Source: CAD feature listing. Evaluate the final solid. Frame: model axes, mm. A direction names the side the tool comes from. Give positions to 0.01 mm unless a question says otherwise; leave off trailing zeros. Write each loop counter-clockwise with the first axis right and the second up, starting at its lowest first coordinate (ties: lowest second). Pieces come first, ordered by that corner, then holes.
```python
from build123d import *

# Parameters (mm, degrees)
F0_W        = 615
F0_H        = 1035
F1_DEPTH    = 436
F2_W        = 383.7750256062
F2_H        = 30
F2_W_2      = 88.2078781724
F3_DEPTH    = 10
F4_W        = 436
F4_H        = 368.6535954475
F5_DEPTH    = 43
F6_T4_DEPTH = 436
F6_T9_DEPTH = 436
F7_W        = 102.6465103626
F7_H        = 30
F7_W_2      = 88.2078781724
F8_DEPTH    = 51
F9_W        = 30
F9_H        = 30
F10_DEPTH   = 55
F11_W       = 30
F11_H       = 30
F12_DEPTH   = 100
F14_DEPTH   = 30
F15_W       = 53
F15_H       = 27.2612595558
F16_DEPTH   = 57
F17_W       = 67.928535223
F17_H       = 25.3568291664
F18_DEPTH   = 81
F20_DEPTH   = 30
F22_DEPTH   = 25


# Not quite as in the source:
# - a fillet or chamfer that OpenCascade refuses, or shapes differently, is made with other operations: its cross-section is extruded or revolved along the edge and cut away or added


with BuildPart() as f1:
    # F0 (on Front) → F1 (new body)
    with BuildSketch(Plane.XZ):
        with Locations((0, 517.5)):
            Rectangle(F0_W, F0_H)
        Polygon((227.5, 80), (-227.5, 80), (-227.5, 360), (-257.5, 360), (-257.5, 440), (-227.5, 440), (-227.5, 520), (-257.5, 520), (-257.5, 665), (-227.5, 665), (-227.5, 955), (227.5, 955), (227.5, 665), (267.5, 665), (297.5, 665), (297.5, 635), (267.5, 635), (267.5, 550), (297.5, 550), (297.5, 520), (267.5, 520), (227.5, 520), (227.5, 440), (297.5, 440), (297.5, 360), (227.5, 360), align=None, mode=Mode.SUBTRACT)
    extrude(amount=F1_DEPTH)

    # F2 (on face) → F3 (cut, through all)
    with BuildSketch(Plane.YZ.offset(307.5)):
        with Locations((-191.8875128031, 535)):
            Rectangle(F2_W, F2_H)
        with Locations((-44.1039390862, 650)):
            Rectangle(F2_W_2, F2_H)
    extrude(amount=-F3_DEPTH, mode=Mode.SUBTRACT)

    # F4 (on face) → F5 (join)
    with BuildSketch(Plane.YZ.offset(307.5)):
        with Locations((-218, 525.7607400417)):
            Rectangle(F4_W, F4_H)
    extrude(amount=F5_DEPTH)

    # F6: chamfer of 45 on 2 edges, made by hand


with BuildPart() as f6_tool2:
    # F6_s3 → F6_t4 (new body)
    with BuildSketch(Plane.XZ):
        Polygon((307.5, 755.0875377655), (352.5, 710.0875377655), (307.5, 710.0875377655), align=None)
    extrude(amount=F6_T4_DEPTH)

    split(bisect_by=Plane.YZ.offset(350.5), keep=Keep.BOTTOM)


with BuildPart() as f1_1:
    add(f1.part)

    # F6_t1: union F6_tool2
    add(f6_tool2.part)


with BuildPart() as f6_tool7:
    # F6_s8 → F6_t9 (new body)
    with BuildSketch(Plane.XZ.offset(436)):
        Polygon((307.5, 296.433942318), (352.5, 341.433942318), (307.5, 341.433942318), align=None)
    extrude(amount=-F6_T9_DEPTH)

    split(bisect_by=Plane.YZ.offset(350.5), keep=Keep.BOTTOM)


with BuildPart() as f1_2:
    add(f1_1.part)

    # F6_t6: union F6_tool7
    add(f6_tool7.part)

    # F7 (on face) → F8 (cut)
    with BuildSketch(Plane.YZ.offset(350.5)):
        with Locations((-384.6767448187, 535)):
            Rectangle(F7_W, F7_H)
        with Locations((-44.1039390862, 650)):
            Rectangle(F7_W_2, F7_H)
    extrude(amount=-F8_DEPTH, mode=Mode.SUBTRACT)

    # F9 (on face) → F10 (join)
    with BuildSketch(Plane.XZ.offset(436)):
        with Locations((282.5, 535)):
            Rectangle(F9_W, F9_H)
    extrude(amount=-F10_DEPTH)

    # F11 (on face) → F12 (join)
    with BuildSketch(Plane.XZ.offset(436)):
        with Locations((282.5, 650)):
            Rectangle(F11_W, F11_H)
    extrude(amount=-F12_DEPTH)

    # F13 (on face) → F14 (join)
    with BuildSketch(Plane.XZ.offset(436)):
        Polygon((227.5, 665), (227.5, 717.9152965546), (-227.5, 717.9152965546), (-227.5, 665), (-257.5, 665), (-257.5, 520), (-227.5, 520), (-227.5, 440), (-257.5, 440), (-257.5, 360), (-227.5, 360), (-227.5, 348.8455712795), (227.5, 348.8455712795), (227.5, 360), (297.5, 360), (297.5, 440), (227.5, 440), (227.5, 520), (267.5, 520), (267.5, 665), align=None)
    extrude(amount=-F14_DEPTH)

    # F15 (on face) → F16 (cut)
    with BuildSketch(Plane(origin=(0, 0, 0), x_dir=(-1, 0, 0), z_dir=(0, 1, 0))):
        with Locations((-324, 426.3693702221)):
            Rectangle(F15_W, F15_H)
    extrude(amount=-F16_DEPTH, mode=Mode.SUBTRACT)

    # F17 (on face) → F18 (cut)
    with BuildSketch(Plane.XZ.offset(436)):
        with Locations((316.5357323885, 373.8530278206)):
            Rectangle(F17_W, F17_H)
    extrude(amount=-F18_DEPTH, mode=Mode.SUBTRACT)

    # F19 (on face) → F20 (join)
    with BuildSketch(Plane(origin=(0, 0, 0), x_dir=(-1, 0, 0), z_dir=(0, 1, 0))):
        Polygon((307.5, 0), (307.5, 348.8455712795), (227.5, 348.8455712795), (227.5, 80), (-227.5, 80), (-227.5, 348.8455712795), (-350.5, 348.8455712795), (-350.5, 339.433942318), (-307.5, 296.433942318), (-307.5, 0), align=None)
        Polygon((-359.9116289616, 348.8455712795), (-350.5, 339.433942318), (-350.5, 348.8455712795), align=None)
        Polygon((-344.6722412109, 717.9152965546), (-227.5, 717.9152965546), (-227.5, 955), (227.5, 955), (227.5, 717.9152965546), (307.5, 717.9152965546), (307.5, 1035), (-307.5, 1035), (-307.5, 755.0875377655), align=None)
    extrude(amount=F20_DEPTH)

    # F21 (on face) → F22 (cut)
    with BuildSketch(Plane.YZ.offset(350.5)):
        Polygon((52.2877275944, 373.7032711506), (0, 373.7032711506), (0, 348.8455712795), (0, 339.433942318), (-23.2749842107, 339.433942318), (-23.2749842107, 317.8108334541), (52.2877275944, 317.8108334541), align=None)
    extrude(amount=F22_DEPTH, mode=Mode.SUBTRACT)


solid = f1_2.part
```
1. Section query B-B (z = 124). Return loops of the section in (x, y), plus the area to 3 significant figures.
2. Line query: probe 1 along Z at (x, y) = (-232.5, -36); probe 2 along Z at (x, y) = (41.5, -317.5); probe 3 along X at (y, z) = (-14, 531.5). Output: solid intervals per line, ascending.
3. Section query D-D (z = 502.5). Return loops of the section in (x, y).
4. Access query for faces 4 (the flat face through (-3, -206, 80)), 5 (the flat face through (287, 15, 717.915)), 6 (the flat face through (263, -200, 360)), 7 (the flat face through (282.571, -421, 374)), 8 (the flat face through (324, -57, 427)). Directions: +Z, -Z, +X, -X, +Y, -Y. A direction counts if a zero-diameter tool reaches every point of the face in a straight line with its end or side. Return the directions, or none.
5. Section query A-A (x = -173.5). Return loops of the section in (y, z).
6. Pin query (flat end, axial travel): P1, Ø8, axis at y = -82.5, z = 875, coming from the +X side; P2, Ø8, axis at x = -126.5, z = 535.5, coming from the +Y side; P3, Ø12, axis at x = 243, y = -279.5, coming from the -Z side; P4, Ø16, axis at x = 334.5, y = -23.5, coming from the +Z side. Return the tip coordinate at first contact, or that it passes through.
7. Pull-direction query (Z, two-part tool) for faces 1 (the flat face through (307.5, -169, 535)), 2 (the flat face through (23, 30, 984)), 3 (the flat face through (297.5, -210, 650)); classes: pulls with the +Z half, pulls with the -Z half, needs draft (parallel to the pull), parting line crosses it, or undercut.
The answers:
1. outline: (-307.5, -436) - (-227.5, -436) - (-227.5, 30) - (-307.5, 30) - close; (227.5, -436) - (307.5, -436) - (307.5, 30) - (227.5, 30) - close
1. area: 74,600 mm2
2. probe 1: z = 0 to 360, 440 to 520, 665 to 1035
2. probe 2: z = 0 to 80, 955 to 1035
2. probe 3: x = -307.5 to -257.5, 307.5 to 350.5
3. outline: (-307.5, -436) - (350.5, -436) - (350.5, 0) - (227.5, 0) - (227.5, -406) - (-227.5, -406) - (-227.5, 0) - (-307.5, 0) - close
4. face 4: +Y, -Y
4. face 5: +X, -X, +Y
4. face 6: +Y
4. face 7: +X, +Y, -Y
4. face 8: +X, +Y
5. outline: (-436, 0) - (30, 0) - (30, 80) - (-436, 80) - close; (-436, 348.85) - (-406, 348.85) - (-406, 717.92) - (-436, 717.92) - close; (-436, 955) - (30, 955) - (30, 1035) - (-436, 1035) - close
6. P1: stops at x = 307.5
6. P2: stops at y = -406
6. P3: stops at z = 0
6. P4: stops at z = 736.09
7. face 1: undercut
7. face 2: needs draft
7. face 3: undercut
